The figure shows three views and two pictorial views of one solid part (mm, origin at its lowest corner). Answer the questions. A direction names the side the tool comes from. Coordinates: 2 decimals unless noted, no trailing zeros. Order: outer loops, then holes, each group sorted by start corner. A loop starts at its lowest first (then second) coordinate and runs counter-clockwise, first axis right, second up. Notation, with made-up numbers: (56, -39.5) -> (108, -39.5) arc R16 cw to (108, -26.5) -> close; hole circle Ø6 at (18, -36). An arc over 180 degrees is marked (long way). Return JSON: item names as keys, results as strings.
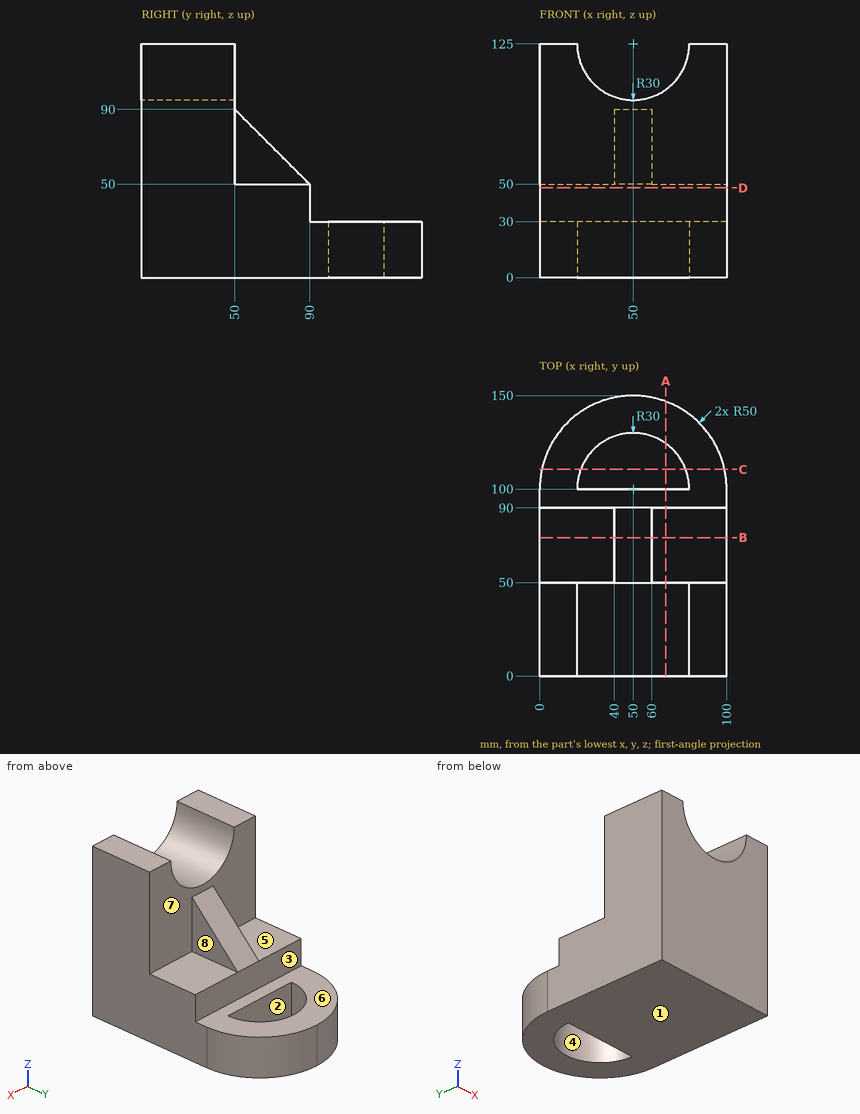
1. Each of these flat-tipped pins is pushed along its axis until it touches: pin 1 Ø10 at (x, z) = (80, 23) entering from +Y; pin 2 Ø16 at (x, z) = (40.5, 40) entering from +Y; pin 3 Ø5 at (x, y) = (64, 33) entering from +Z (3 decimals). Where does it stop, or does it pass through?
Answer block:
{"pin 1": "stops at y = 143.3", "pin 2": "stops at y = 90", "pin 3": "stops at z = 99.945"}
2. Consider line 1 (Y direction, x = 61.5, z = 77); line 2 (Z direction, x = 57.5, y = 130). Determine where each line is inside the solid, lowest interval first. Write a range as from..to.
Answer block:
{"line 1": "y = 0..50", "line 2": "z = 0..30"}
3. For the marked faces 4, 5, 6, 7 and 8, determine the directions among +Z, -Z, +X, -X, +Y, -Y from which every point of the face is accessible in a straight line to the end or side of a thin tool.
Answer block:
{"face 4": "+Z, -Z", "face 5": "+Z, -X, +Y", "face 6": "+Z, +X, -X, +Y", "face 7": "+Z, +Y", "face 8": "+Z, +X, +Y"}
4. Determine the mould class of the marked faces 1, 2 and 3 for opening direction Y: pulls with the +Y half, pulls with the -Y half, needs draft (parallel to the pull), parting line crosses it, or undercut.
Answer block:
{"face 1": "needs draft", "face 2": "undercut", "face 3": "pulls with the +Y half"}
5. The part is cut by section C-C on y = 110.5. Give the vertices of the cut face in (x, z) (1 decimal), and give its area (3 significant figures).
Answer block:
{"outline": "(1.1, 0) -> (21.9, 0) -> (21.9, 30) -> (1.1, 30) -> close; (78.1, 0) -> (98.9, 0) -> (98.9, 30) -> (78.1, 30) -> close", "area": "1,250 mm2"}
6. The part is cut by section B-B on y = 74. Give the vertices of the cut face in (x, z), and give its area (3 significant figures).
Answer block:
{"outline": "(0, 0) -> (100, 0) -> (100, 50) -> (60, 50) -> (60, 66) -> (40, 66) -> (40, 50) -> (0, 50) -> close", "area": "5,320 mm2"}
7. The part is cut by section A-A on x = 67.5. Give the vertices of the cut face in (y, z).
Answer block:
{"outline": "(0, 0) -> (100, 0) -> (100, 30) -> (90, 30) -> (90, 50) -> (50, 50) -> (50, 100.63) -> (0, 100.63) -> close; (124.37, 0) -> (146.84, 0) -> (146.84, 30) -> (124.37, 30) -> close"}
8. The part is cut by section D-D on z = 48. Give the vertices of the cut face in (x, y), and give its area (3 significant figures).
Answer block:
{"outline": "(0, 0) -> (100, 0) -> (100, 90) -> (0, 90) -> close", "area": "9,000 mm2"}
